For this review, take the finished solid that the model builds, in its own axes (mm). Face numbers are marked on the shaded views. Round coordinates to 2 decimals unless told otherwise and drop trailing zeros. Order: outer loops, then holes, each group sorted by start corner. A loop starts at its lowest first (then second) coordinate and runs counter-clockwise, first axis right, second up. Notation, with made-up numbers: (70.25, 40) -> (99.25, 40) arc R18 cw to (99.25, 56) -> close; hole circle Ø3 at (63.25, 70.5). An arc over 180 degrees is marked (long way). Use a Markdown table: item, result. Add a question column.
1) Draft analysis for pull direction Z (two halves, no side actions). For the marked faces 1 and 2, state which applies: pulls with the +Z half, pulls with the -Z half, needs draft (parallel to the pull), parting line crosses it, or undercut.
2) Wall thickness on line 1 along Z through (x, y) = (0, -1.1); line 2 along X through (y, z) = (-0.7, -1); line 3 along Z through (x, y) = (1, -0.25): over which ranges is each line inside the solid? List them lowest first. Write a range as [from, to].
3) Consider section C-C (y = -0.9). State the section outline as (x, z) points.
4) Clearance check with a flat-ended pin moving along its axis: P1, Ø1, axis at x = 1, z = -1, coming from the -Y side. State where the tip first meets the part, or that it passes through.
5) Consider section D-D (y = -0.15). State the section outline as (x, z) points, plus the area to 3 significant figures.
```python
from build123d import *

# Parameters (mm, degrees)
F0_R     = 3.5
F0_R_2   = 2.5
F1_DEPTH = 2
F2_R     = 0.5
F3_SIZE  = 0.49999


# Not quite as in the source:
# - a fillet or chamfer is up to 0.001 mm smaller than in the source, because OpenCascade refuses the exact size


with BuildPart() as f1:
    # F0 (on Front) → F1 (new body)
    with BuildSketch(Plane.XZ):
        Circle(F0_R)
        Circle(F0_R_2, mode=Mode.SUBTRACT)
    extrude(amount=F1_DEPTH)

    # F2
    f2_edges = [f1.edges().sort_by_distance(p)[0] for p in [
        (-3.5, -2, 0),
        (3.5, -1, 0),
        (-3.5, 0, 0),
    ]]
    fillet(f2_edges, radius=F2_R)

    # F3 (size 0.5 in the source; OpenCascade refuses exactly that, so slightly less here)
    f3_edges = [f1.edges().sort_by_distance(p)[0] for p in [
        (-2.5, -2, 0),
        (-2.5, 0, 0),
    ]]
    chamfer(f3_edges, length=F3_SIZE)


solid = f1.part
```
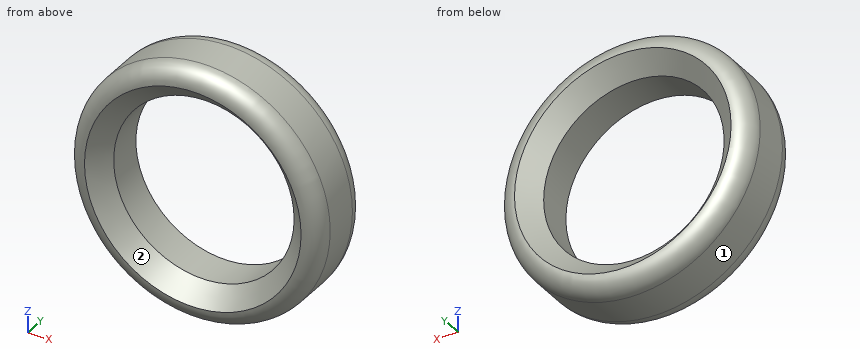
Results list:
| question | item | result |
|---|---|---|
| 1 | face 1 | parting line crosses it |
| 1 | face 2 | undercut |
| 2 | line 1 | [-3.5, -2.5], [2.5, 3.5] |
| 2 | line 2 | [-3.35, -2.29], [2.29, 3.35] |
| 2 | line 3 | [-3.28, -2.56], [2.56, 3.28] |
| 3 | outline | circle Ø7 at (0, 0); hole circle Ø5 at (0, 0) |
| 4 | P1 | through |
| 5 | outline | circle Ø6.71 at (0, 0); hole circle Ø5.7 at (0, 0) |
| 5 | area | 9.89 mm2 |
